Here's how the part is built. I have some questions about the finished solid (model axes, mm). A direction names the side the tool comes from. Coordinates: 2 decimals unless noted, no trailing zeros. Write each loop counter-clockwise with the first axis right and the second up, starting at its lowest first coordinate (ties: lowest second). Pieces come first, ordered by that corner, then holes.
Item 1: For faces 1 (the face through (-0.203, 1.617, 0.67)), 2 (the face through (22, 0, 1)), which set-ups out of +Z, -Z, +X, -X, +Y, -Y let a thin tool reach every point of the face, with its end or its side?
Item 2: Please list where these lines run through material, in increasing order: line 1 (Z direction, x = 42, y = 0.05); line 2 (Y direction, x = 5.5, z = 0.3); line 3 (X direction, y = 1.15, z = 1).
Item 3: I'm going to push flat-ended pins straight in: P1, Ø2, axis at x = 36.5, y = -1, coming from the -Z side; P2, Ø1.5, axis at x = 10.5, z = 0.5, coming from the +Y side. Where does each tip first touch, or does it pass through?
Item 4: I want a section at A-A (x = 14). Please give me the cut outline in (y, z), and give its area (3 significant figures).
Autodesk Inventor part; units mm, degrees
ref_plane "Work Plane1" through (29, 0, 0) normal (0, -1, 0) x (1, 0, 0)
ref_plane "YZ Plane" through (0, 0, 0) normal (1, 0, 0) x (0, 1, 0)
ref_plane "XZ Plane" through (0, 0, 0) normal (0, 1, 0) x (-1, 0, 0)
sketch "Sketch1" plane through (0, 0, 0) normal (0, 0, 1) x (1, 0, 0)
  line L0 (-0.0833, 0) -> (45, 0)
  line L1 (45, 0) -> (45, 1)
  line L2 (45, 1) -> (42, 1)
  line L3 (42, 1) -> (41.6932, 1)
  line L4 (41.6932, 1) -> (0, 1)
  line L5 (0, 1) -> (0, 1.75)
  line L6 (0, 1.75) -> (-1.2, 1.75)
  line L7 (-1.2, 1.75) -> (-1.2, 0.7217)
  line L8 (-1.2, 0.7217) -> (-0.5, 0.7217)
  line L9 (-0.5, 0.7217) -> (-0.0833, 0)
  line L10 (-10.44, 0) -> (54.24, 0)
  line L11 (0, -0.35) -> (0, 2.1)
  line L12 (42, 1) -> (0, 1) construction
  dimension "d1" = 3
  dimension "d2" = 0.3068
  dimension "d3" = 1.2
  dimension "d4" = 0.7
  dimension "d5" = 60
  dimension "d6" = 2
  dimension "d7" = 2
  dimension "d8" = 1.4434
  dimension "d9" = 3.5
  dimension "d26" = 45
revolve "Body" add sketch "Sketch1" angle 360 about axis through (-0.0833, 0, 0) along (1, 0, 0)
sketch "Sketch2" plane through (-1.2, 0, 0) normal (-1, 0, 0) x (0, 0, 1)
  circle A0 centre (0, 0) radius 0.7217
  line L0 (0, -2.45) -> (0, 2.45)
  line L1 (-2.45, 0) -> (2.45, 0)
  line L2 (0.7217, 0) -> (0.3608, -0.625)
  line L3 (0.3608, -0.625) -> (-0.3608, -0.625)
  line L4 (-0.3608, -0.625) -> (-0.7217, 0)
  line L5 (-0.7217, 0) -> (-0.3608, 0.625)
  line L6 (-0.3608, 0.625) -> (0.3608, 0.625)
  line L7 (0.3608, 0.625) -> (0.7217, 0)
extrude "Slot" add sketch "Sketch2" against normal up to next contours L7 A0 | A0 L2 | L6 L0 A0 | A0 L0 L3 | L0 L6 A0 | A0 L3 L0 | L4 A0 | A0 L5
fillet "Fillet1" radius 0.8 1 edges at (-1.2, -1.75, 0)
chamfer "Chamfer1" distance 0.3067 distance2 0.3067 1 edges at (45, -1, 0) measured on face at (45, -0.2495, -0.4023)
ref_plane "Work Plane1" through (29, 0, 0) normal (0, -1, 0) x (1, 0, 0)
fillet "Fillet2" radius 0.1 1 edges at (0, -1, 0)
thread "Thread2"
equation "\"d15\" = -0.5 * SPD + 0.5 * GD"
equation "\"d16\" = GUL"
equation "\"GD\" = NND"
equation "\"NLG\" = 6"
equation "\"GEL\" = 4.5"
equation "\"KOD\" = 5.7"
equation "\"KOH\" = 1.65"
equation "\"INTI\" = 1.04"
equation "\"GAL\" = 0.61345 * PTC"
equation "\"GUL\" = 0.61345 * PTC"
equation "\"BDM\" = NND"
equation "\"SW\" = 2"
equation "\"RR\" = 1.45"
equation "\"SPD\" = NND - 1.2269 * PTC"
equation "\"R\" = 0.3"
equation "\"TOA\" = 30deg"
equation "\"GD1\" = THREADDIA - 1.2269 * PTC"
equation "\"THREADDIA\" = 3"
equation "\"PTC\" = 0.5"
equation "\"NND\" = 3"
equation "\"KOH1\" = 0.2"
equation "\"E0\" = 2.303"
properties part number "M2x35 Bolt" material "Stainless Steel"
Answer:
1. face 1: +X, -X
1. face 2: +X
2. line 1: z = -1 to 1
2. line 2: y = -0.95 to 0.95
2. line 3: x = -0.96 to 0
3. P1: stops at z = -1
3. P2: stops at y = 1
4. outline: circle Ø2 at (0, 0)
4. area: 3.14 mm2
